Verification items for the finished model (mm, model axes). Face numbers are marked on the shaded views. A direction names the side the tool comes from. Coordinates: 2 decimals unless noted, no trailing zeros. Write each loop counter-clockwise with the first axis right and the second up, starting at its lowest first coordinate (ties: lowest second). Pieces come first, ordered by that corner, then holes.
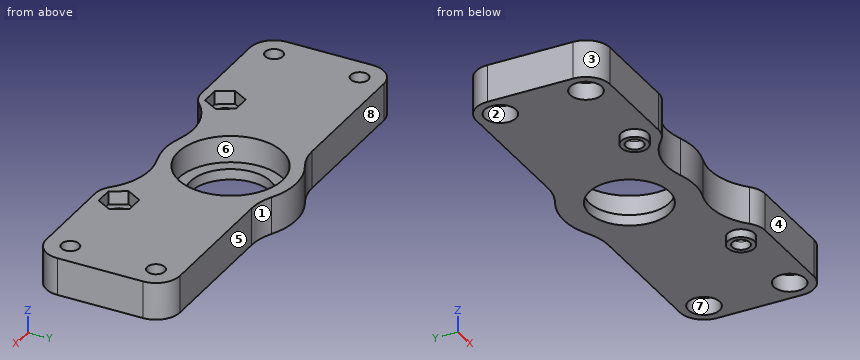
```python
from build123d import *

# Parameters (mm, degrees)
SKETCH1_R           = 9.75
SKETCH1_R_2         = 1.65
BOSS_EXTRUDE1_DEPTH = 7
FILLET1_R           = 10
SKETCH2_R           = 9.75
SKETCH2_R_2         = 7.5
BOSS_EXTRUDE2_DEPTH = 2
CUT_EXTRUDE1_DEPTH  = 2.5
SKETCH4_R           = 2.5
SKETCH4_R_2         = 1.65
BOSS_EXTRUDE3_DEPTH = 1.5
SKETCH5_R           = 2.95
CUT_EXTRUDE2_DEPTH  = 3.2


with BuildPart() as part:
    # Sketch1 → Boss-Extrude1 (new body)
    with BuildSketch(Plane.XY):
        with BuildLine():
            Line((-35.5, 9.588593938), (-7.623737029, 9.588593938))
            ThreePointArc((-7.623737029, 9.588593938), (0, 12.25), (7.623737029, 9.588593938))
            Line((7.623737029, 9.588593938), (35.5, 9.588593938))
            ThreePointArc((35.5, 9.588593938), (38.681980515, 8.270574454), (40, 5.088593938))
            Line((40, 5.088593938), (40, -10.911406062))
            ThreePointArc((40, -10.911406062), (38.681980515, -14.093386577), (35.5, -15.411406062))
            Line((35.5, -15.411406062), (18.542115282, -15.411406062))
            ThreePointArc((18.542115282, -15.411406062), (16.87570332, -15.091486345), (15.44623271, -14.177215472))
            ThreePointArc((15.44623271, -14.177215472), (10.021005103, -11.295196388), (3.88623271, -11.617215472))
            ThreePointArc((3.88623271, -11.617215472), (0, -12.25), (-3.88623271, -11.617215472))
            ThreePointArc((-3.88623271, -11.617215472), (-10.021005103, -11.295196388), (-15.44623271, -14.177215472))
            ThreePointArc((-15.44623271, -14.177215472), (-16.87570332, -15.091486345), (-18.542115282, -15.411406062))
            Line((-18.542115282, -15.411406062), (-35.5, -15.411406062))
            ThreePointArc((-35.5, -15.411406062), (-38.681980515, -14.093386577), (-40, -10.911406062))
            Line((-40, -10.911406062), (-40, 5.088593938))
            ThreePointArc((-40, 5.088593938), (-38.681980515, 8.270574454), (-35.5, 9.588593938))
        make_face()
        Circle(SKETCH1_R, mode=Mode.SUBTRACT)
        with Locations((-35.5, 5.088593938)):
            Circle(SKETCH1_R_2, mode=Mode.SUBTRACT)
        with Locations((35.5, 5.088593938)):
            Circle(SKETCH1_R_2, mode=Mode.SUBTRACT)
        with Locations((-18.542115282, -10.911406062)):
            Circle(SKETCH1_R_2, mode=Mode.SUBTRACT)
        with Locations((-35.5, -10.911406062)):
            Circle(SKETCH1_R_2, mode=Mode.SUBTRACT)
        with Locations((18.542115282, -10.911406062)):
            Circle(SKETCH1_R_2, mode=Mode.SUBTRACT)
        with Locations((35.5, -10.911406062)):
            Circle(SKETCH1_R_2, mode=Mode.SUBTRACT)
    extrude(amount=BOSS_EXTRUDE1_DEPTH)

    # Fillet1
    fillet1_edges = [part.edges().sort_by_distance(p)[0] for p in [
        (-7.623737029, 9.588593938, 3.5),
        (7.623737029, 9.588593938, 3.5),
    ]]
    fillet(fillet1_edges, radius=FILLET1_R)

    # Sketch2 → Boss-Extrude2 (add)
    with BuildSketch(Plane.XY):
        Circle(SKETCH2_R)
        Circle(SKETCH2_R_2, mode=Mode.SUBTRACT)
    extrude(amount=BOSS_EXTRUDE2_DEPTH)

    # Sketch3 → Cut-Extrude1 (cut)
    with BuildSketch(Plane.XY.offset(7)):
        Polygon((-16.867799501, -8.011406062), (-20.216431062, -8.011406062), (-21.890746843, -10.911406062), (-20.216431062, -13.811406062), (-16.867799501, -13.811406062), (-15.19348372, -10.911406062), align=None)
        Polygon((20.216431062, -8.011406062), (16.867799501, -8.011406062), (15.19348372, -10.911406062), (16.867799501, -13.811406062), (20.216431062, -13.811406062), (21.890746843, -10.911406062), align=None)
    extrude(amount=-CUT_EXTRUDE1_DEPTH, mode=Mode.SUBTRACT)

    # Sketch4 → Boss-Extrude3 (add)
    with BuildSketch(Plane(origin=(0, 0, 0), x_dir=(-1, 0, 0), z_dir=(0, 0, -1))):
        with Locations((-18.542115282, -10.911406062)):
            Circle(SKETCH4_R)
        with Locations((-18.542115282, -10.911406062)):
            Circle(SKETCH4_R_2, mode=Mode.SUBTRACT)
        with Locations((18.542115282, -10.911406062)):
            Circle(SKETCH4_R)
        with Locations((18.542115282, -10.911406062)):
            Circle(SKETCH4_R_2, mode=Mode.SUBTRACT)
    extrude(amount=BOSS_EXTRUDE3_DEPTH)

    # Sketch5 → Cut-Extrude2 (cut)
    with BuildSketch(Plane(origin=(0, 0, 0), x_dir=(-1, 0, 0), z_dir=(0, 0, -1))):
        with Locations((-35.5, 5.088593938)):
            Circle(SKETCH5_R)
        with Locations((-35.5, -10.911406062)):
            Circle(SKETCH5_R)
        with Locations((35.5, 5.088593938)):
            Circle(SKETCH5_R)
        with Locations((35.5, -10.911406062)):
            Circle(SKETCH5_R)
    extrude(amount=-CUT_EXTRUDE2_DEPTH, mode=Mode.SUBTRACT)


solid = part.part
```
1. Sectioned sample at D-D, the plane x = -26.5. Record the boundary of the cut face in (y, z).
2. Material ranges on L1, parallel to Y at x = -35.5, z = 6.05; L2, parallel to Y at x = -35.5, z = 1.6; L3, parallel to Y at x = 0, z = 1.1, recorded low to high.
3. Draft check along X on the marked faces 1, 2, 3 and 4. Enter one of: pulls with the +X half, pulls with the -X half, needs draft (parallel to the pull), parting line crosses it, or undercut.
4. Gauge pin test, flat ends, axial feed: P1, Ø7.5, axis at x = 35.5, y = 5.09, coming from the -Z side; P2, Ø5, axis at x = 6, z = 2.5, coming from the -Y side; P3, Ø4.5, axis at x = 35.5, y = -10.5, coming from the -Z side. Record the tip position at first contact, or that the pin passes through.
5. Tool access check on the marked faces 5, 6, 7 and 8. Record the directions out of +Z, -Z, +X, -X, +Y, -Y that give a thin tool (end or side, any length) a straight path to the whole face; none if there is none.
6. Sectioned sample at A-A, the plane x = 0. Record the boundary of the cut face in (y, z), and give its area (3 significant figures).
7. Sectioned sample at B-B, the plane y = -1.25. Record the boundary of the cut face in (x, z), and give its area (3 significant figures).
8. Sectioned sample at C-C, the plane z = 6.25. Give the number of separate pieces and of enclosed holes in the cut face, and give its area (3 significant figures).
Outcome:
1. outline: (-15.41, 0) - (9.59, 0) - (9.59, 7) - (-15.41, 7) - close
2. L1: y = -15.41 to -12.56, -9.26 to 3.44, 6.74 to 9.59
2. L2: y = -15.41 to -13.86, -7.96 to 2.14, 8.04 to 9.59
2. L3: y = -12.25 to -7.5, 7.5 to 12.25
3. face 1: pulls with the +X half
3. face 2: undercut
3. face 3: pulls with the -X half
3. face 4: needs draft
4. P1: stops at z = 0
4. P2: stops at y = -11.74
4. P3: stops at z = 3.2
5. face 5: +Z, -Z, +X, +Y
5. face 6: +Z
5. face 7: -Z
5. face 8: +Z, -Z, -X, +Y
6. outline: (-12.25, 0) - (-7.5, 0) - (-7.5, 2) - (-9.75, 2) - (-9.75, 7) - (-12.25, 7) - close; (7.5, 0) - (12.25, 0) - (12.25, 7) - (9.75, 7) - (9.75, 2) - (7.5, 2) - close
6. area: 44.0 mm2
7. outline: (-40, 0) - (-7.4, 0) - (-7.4, 2) - (-9.67, 2) - (-9.67, 7) - (-40, 7) - close; (7.4, 0) - (40, 0) - (40, 7) - (9.67, 7) - (9.67, 2) - (7.4, 2) - close
7. area: 434 mm2
8. separate pieces: 1
8. enclosed holes: 7
8. area: 1,510 mm2
